Geometry check sheet. Reference: the model listing, model coordinates, mm. Face numbers are marked on the shaded views. A direction names the side the tool comes from. Round coordinates to 2 decimals unless told otherwise and drop trailing zeros. Write each loop counter-clockwise with the first axis right and the second up, starting at its lowest first coordinate (ties: lowest second). Pieces come first, ordered by that corner, then holes. Notation, with made-up numbers: (-23.5, 5) -> (14.5, 5) arc R30 cw to (14.5, 30) -> close; hole circle Ø4 at (41.5, -18). An arc over 180 degrees is marked (long way). One line per question, with ' | ' between items.
```python
from build123d import *

# Parameters (mm, degrees)
CYLINDER_R        = 15
CYLINDER_DEPTH    = 4
CYLINDER002_R     = 8
CYLINDER002_DEPTH = 5
CYLINDER003_R     = 4.2
CYLINDER003_DEPTH = 10
CHAMFER_SIZE      = 1
CHAMFER001_SIZE   = 1


with BuildPart() as part:
    # Cylinder → Cylinder (join)
    with BuildSketch(Plane.XY):
        Circle(CYLINDER_R)
    extrude(amount=CYLINDER_DEPTH)

    # Cylinder002 → Cylinder002 (join)
    with BuildSketch(Plane.XY):
        Circle(CYLINDER002_R)
    extrude(amount=CYLINDER002_DEPTH)

    # Cylinder003 → Cylinder003 (cut)
    with BuildSketch(Plane.XY):
        Circle(CYLINDER003_R)
    extrude(amount=CYLINDER003_DEPTH, mode=Mode.SUBTRACT)

    # Chamfer
    chamfer_edges = [part.edges().sort_by_distance(p)[0] for p in [
        (-15, 0, 4),
        (15, 0, 2),
        (-15, 0, 0),
    ]]
    chamfer(chamfer_edges, length=CHAMFER_SIZE)

    # Chamfer001
    chamfer001_edges = [part.edges().sort_by_distance(p)[0] for p in [
        (-4.2, 0, 5),
        (4.2, 0, 2.5),
        (-4.2, 0, 0),
    ]]
    chamfer(chamfer001_edges, length=CHAMFER001_SIZE)


solid = part.part
```
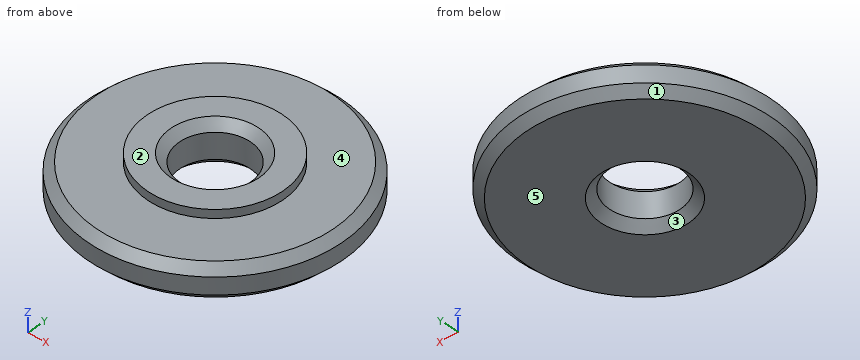
(1) Sectioned sample at D-D on z = 0.4. Record the cut outline in (x, y).
Resolved:
outline: circle Ø28.8 at (0, 0); hole circle Ø9.6 at (0, 0)
(2) Sectioned sample at A-A on x = 0. Record the cut outline in (y, z).
Resolved:
outline: (-15, 1) -> (-14, 0) -> (-5.2, 0) -> (-4.2, 1) -> (-4.2, 4) -> (-5.2, 5) -> (-8, 5) -> (-8, 4) -> (-14, 4) -> (-15, 3) -> close; (4.2, 1) -> (5.2, 0) -> (14, 0) -> (15, 1) -> (15, 3) -> (14, 4) -> (8, 4) -> (8, 5) -> (5.2, 5) -> (4.2, 4) -> close
(3) Draft check along Y on the marked faces 1, 2 and 3. Enter one of: +Y half, -Y half, draft (parallel to the pull), parting line (faces both ways), or undercut.
Resolved:
face 1: parting line | face 2: draft | face 3: undercut
(4) Go/stop test with flat-tipped pins: pin 1 (2 mm diameter, centred on x = -9, z = 4.5, fed in from +Y); pin 2 (2 mm diameter, centred on x = 10, z = 2, fed in from +Y); pin 3 (2 mm diameter, centred on y = 7.5, z = 2.5, fed in from -X). Record where each tip stops, or that it passes through.
Resolved:
pin 1: stops at y = 11.58 | pin 2: stops at y = 12 | pin 3: stops at x = -13.52
(5) Material ranges on line 1 (Y direction, x = 0, z = 1.9); line 2 (Z direction, x = -4.25, y = 10.5); line 3 (Y direction, x = -2.25, z = 4.7), recorded low to high.
Resolved:
line 1: y = -15 to -4.2, 4.2 to 15 | line 2: z = 0 to 4 | line 3: y = -7.68 to -4.35, 4.35 to 7.68
(6) Access from +Z, -Z, +X, -X, +Y, -Y to the whole of each face (thin tool, end or side, straight path). Record for the marked faces 4 and 5.
Resolved:
face 4: +Z | face 5: -Z, +X, -X, +Y, -Y
(7) Sectioned sample at C-C on z = 3.4. Record the cut outline in (x, y), then the cut area to 3 significant figures.
Resolved:
outline: circle Ø29.2 at (0, 0); hole circle Ø8.4 at (0, 0) | area: 614 mm2
